```python
from build123d import *

# Parameters (mm, degrees)
BOSS_CONFIGUP_DEPTH       = 9.525
SKETCH2_W                 = 4.7625
SKETCH2_H                 = 9.525
CUT_NUTSLOT_DEPTH         = 1.5875
F_2_CLEARANCE_HOLE1_D     = 2.4384
F_2_CLEARANCE_HOLE1_DEPTH = 1.5875


with BuildPart() as part:
    # Sketch-ConfigUp → Boss-ConfigUp (new body)
    with BuildSketch(Plane.XY):
        with BuildLine():
            Line((7.315587682, 2.213714366), (7.104153068, 1.103671392))
            ThreePointArc((7.104153068, 1.103671392), (7.02887285, 0.587148983), (6.557966762, 0.361960248))
            Line((6.557966762, 0.361960248), (5.304651863, -0.305823275))
            Line((5.304651863, -0.305823275), (-6.711147083, -0.305823275))
            Line((-6.711147083, -0.305823275), (-6.711147083, -3.480823275))
            Line((-6.711147083, -3.480823275), (15.578632688, -3.480823275))
            Line((15.578632688, -3.480823275), (15.578632688, 0.0709065))
            Line((15.578632688, 0.0709065), (11.489555896, 4.360169677))
            ThreePointArc((11.489555896, 4.360169677), (11.115827658, 4.815287007), (11.286259089, 5.378987021))
            Line((11.286259089, 5.378987021), (12.499382227, 11.378887869))
            ThreePointArc((12.499382227, 11.378887869), (12.108389527, 11.968060772), (11.519216625, 11.577068073))
            Line((11.519216625, 11.577068073), (10.575379996, 6.90901253))
            Line((10.575379996, 6.90901253), (8.002147984, 5.265295329))
            Line((8.002147984, 5.265295329), (5.000864154, 21.195713966))
            ThreePointArc((5.000864154, 21.195713966), (5.515878545, 21.515221814), (5.923633344, 21.963620199))
            ThreePointArc((5.923633344, 21.963620199), (5.792717863, 22.658502302), (5.09783576, 22.527586821))
            ThreePointArc((5.09783576, 22.527586821), (3.870546529, 22.033736006), (2.944624614, 22.978614881))
            ThreePointArc((2.944624614, 22.978614881), (2.360697542, 23.377399504), (1.96191292, 22.793472432))
            ThreePointArc((1.96191292, 22.793472432), (2.679570384, 21.54396233), (4.01815246, 21.010571517))
            Line((4.01815246, 21.010571517), (7.116284258, 4.566096638))
            ThreePointArc((7.116284258, 4.566096638), (7.329390516, 4.240581461), (7.710370279, 4.161658542))
            ThreePointArc((7.710370279, 4.161658542), (7.941736771, 4.080744656), (7.986384484, 3.83973824))
            ThreePointArc((7.986384484, 3.83973824), (7.67084838, 3.018532349), (7.315587682, 2.213714366))
        make_face()
        with BuildLine():
            Line((13.528041298, -0.305823275), (7.778926955, -0.305823275))
            ThreePointArc((7.778926955, -0.305823275), (7.581920737, -1.036684597), (7.028198014, -0.520582992))
            ThreePointArc((7.028198014, -0.520582992), (7.40177857, 0.312546128), (8.086491983, 0.916561115))
            Line((8.086491983, 0.916561115), (8.297926597, 2.026604089))
            ThreePointArc((8.297926597, 2.026604089), (8.15636952, 2.899078498), (9.028843929, 3.040635574))
            ThreePointArc((9.028843929, 3.040635574), (9.1929804, 3.047421198), (9.225253016, 3.208496658))
            Line((9.225253016, 3.208496658), (8.538827812, 4.566096638))
            ThreePointArc((8.538827812, 4.566096638), (8.51473614, 4.804983129), (8.657105129, 4.998317646))
            Line((8.657105129, 4.998317646), (9.788823733, 5.721231603))
            ThreePointArc((9.788823733, 5.721231603), (10.079629218, 5.764709454), (10.306093487, 5.577167225))
            ThreePointArc((10.306093487, 5.577167225), (10.642479335, 4.649344509), (10.765760559, 3.670154961))
            Line((10.765760559, 3.670154961), (13.32194446, 0.988829556))
            Line((13.32194446, 0.988829556), (14.12753679, 0.143798344))
            ThreePointArc((14.12753679, 0.143798344), (14.352707563, -0.780903824), (13.528041298, -0.305823275))
        make_face(mode=Mode.SUBTRACT)
    extrude(amount=BOSS_CONFIGUP_DEPTH)

    # Sketch2 → Cut-NutSlot (cut)
    with BuildSketch(Plane(origin=(0.004306068, -0.305823275, 0), x_dir=(-1, 0, 0), z_dir=(0, -1, 0))):
        with Locations((-10.649178058, -4.7625)):
            Rectangle(SKETCH2_W, SKETCH2_H)
        with Locations((1.159203152, -4.7625)):
            Rectangle(SKETCH2_W, SKETCH2_H)
    extrude(amount=CUT_NUTSLOT_DEPTH, mode=Mode.SUBTRACT)

    # #2 Clearance Hole1
    with Locations(Plane(origin=(0, -3.480823275, 0), x_dir=(-1, 0, 0), z_dir=(0, -1, 0))):
        with Locations((-10.653484126, -4.7625), (1.154897083, -4.7625)):
            Hole(F_2_CLEARANCE_HOLE1_D / 2, depth=F_2_CLEARANCE_HOLE1_DEPTH)


solid = part.part
```
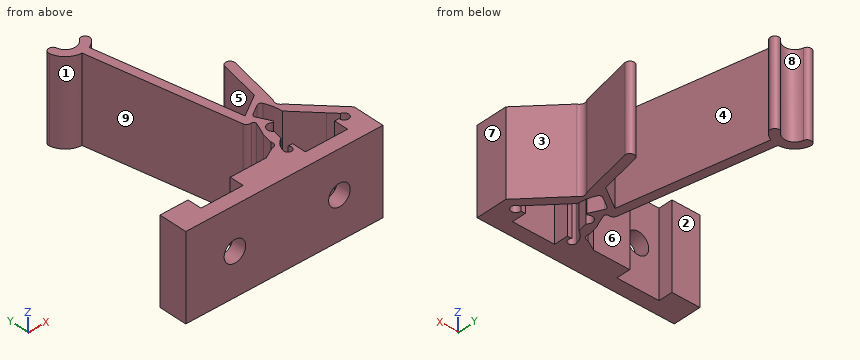
Geometry: final body of the model. Coordinates: model frame, mm. Face numbers are marked on the shaded views. A direction names the side the tool comes from. Round coordinates to 2 decimals unless told otherwise and drop trailing zeros. Write each loop counter-clockwise with the first axis right and the second up, starting at its lowest first coordinate (ties: lowest second). Pieces come first, ordered by that corner, then holes.
Item 1: Pin query (flat end, axial travel): P1, Ø5, axis at x = 13, z = 2.5, coming from the +Y side; P2, Ø1.4, axis at x = -1.5, z = 5.5, coming from the +Y side; P3, Ø2.5, axis at x = -4.5, z = 6, coming from the +Y side. Return the tip coordinate at first contact, or that it passes through.
Item 2: Section query A-A (y = -1.5). Return loops of the section in (x, z) (3 decimals), plus the area to 3 significant figures.
Item 3: Mould query, pull axis X, two halves, no side actions, for the marked faces 6, 7, 8 and 9. Classes: +X half, -X half, draft (parallel to the pull), parting line (faces both ways), or undercut.
Item 4: Set-up query: the marked faces 1, 2, 3, 4 and 5. Return all of +Z, -Z, +X, -X, +Y, -Y with unobstructed straight access to the full face (end or side cutting, diameter ignored); none if empty.
Item 5: Section query C-C (y = 7.5). Return loops of the section in (x, z) (3 decimals).
Item 6: Section query B-B (x = -0.5). Return loops of the section in (y, z) (3 decimals).
Item 7: Section query D-D (x = -4.75). Return loops of the section in (y, z) (3 decimals).
Item 8: Material intervals for L1, parallel to Y at x = -1, z = 1; L2, parallel to X at y = -0.5, z = 8.25; L3, parallel to Z at x = 10.25, y = -2.5 (3 decimals), sorted ascending.
Completed:
1. P1: stops at y = 11.98
1. P2: stops at y = -1.89
1. P3: stops at y = -0.31
2. outline: (-6.711, 0) - (-3.536, 0) - (-3.536, 9.525) - (-6.711, 9.525) - close; (1.226, 0) - (8.272, 0) - (8.272, 9.525) - (1.226, 9.525) - close; (13.035, 0) - (15.579, 0) - (15.579, 9.525) - (13.035, 9.525) - close
2. area: 122 mm2
3. face 6: draft
3. face 7: +X half
3. face 8: undercut
3. face 9: -X half
4. face 1: +Z, -Z, -X
4. face 2: +Z, -Z, -X, +Y
4. face 3: +Z, -Z, +X
4. face 4: +Z, -Z
4. face 5: +Z, -Z, +Y
5. outline: (6.564, 0) - (7.581, 0) - (7.581, 9.525) - (6.564, 9.525) - close; (10.695, 0) - (11.715, 0) - (11.715, 9.525) - (10.695, 9.525) - close
6. outline: (-3.481, 0) - (-1.893, 0) - (-1.893, 3.734) - (-3.481, 3.734) - close; (-3.481, 5.791) - (-1.893, 5.791) - (-1.893, 9.525) - (-3.481, 9.525) - close
7. outline: (-3.481, 0) - (-0.306, 0) - (-0.306, 9.525) - (-3.481, 9.525) - close
8. L1: y = -3.48 to -1.89
8. L2: x = -6.71 to -3.54, 1.23 to 7.03, 7.89 to 8.27, 13.03 to 13.54, 14.54 to 15.58
8. L3: z = 0 to 3.612, 5.913 to 9.525
